Part model, mm, in its own coordinate system. Give positions to 0.01 mm unless a question says otherwise; leave off trailing zeros. Order: outer loops, then holes, each group sorted by start corner. A loop starts at its lowest first (then second) coordinate and runs counter-clockwise, first axis right, second up.
1. Slice it at A-A on y = 44.45. List the corners of the cut face in (x, z).
2. Slice it at C-C on z = 11. Give the number of separate pieces and of enclosed holes in the cut face, and give its area (3 significant figures).
3. Probe line 1 (Y direction, x = 44.45, z = 3.75); line 2 (Y direction, x = 25.4, z = 7.75); line 3 (Y direction, x = 46, z = 6.25). List the from-to ranges inside material, lowest first.
4. Slice it at B-B on x = 25.4. List the corners of the cut face in (y, z), and give its area (3 significant figures).
5. Mould opens along Y. For faces 1 (the cylindrical face through (17.375, 6.424, 6.439)), 2 (the flat face through (0, 25, 6)), 3 (the flat face through (25, 0, 6)) say: +Y half, -Y half, draft (parallel to the pull), parting line (faces both ways), or undercut.
from build123d import *

# Parameters (mm, degrees)
SKETCH1_W           = 50.8
SKETCH1_H           = 50.8
BOSS_EXTRUDE1_DEPTH = 12.7
SKETCH2_R           = 7.62
CUT_EXTRUDE1_DEPTH  = 13.7
SKETCH3_R           = 4.064
CUT_EXTRUDE2_DEPTH  = 13.7
SKETCH4_R           = 1.6764
CUT_EXTRUDE3_DEPTH  = 13.7


with BuildPart() as part:
    # Sketch1 → Boss-Extrude1 (new body)
    with BuildSketch(Plane.XY):
        with Locations((25.4, 25.4)):
            Rectangle(SKETCH1_W, SKETCH1_H)
    extrude(amount=BOSS_EXTRUDE1_DEPTH)

    # Sketch2 → Cut-Extrude1 (cut, through all)
    with BuildSketch(Plane.XY.offset(12.7)):
        with Locations((25.4, 25.4)):
            Circle(SKETCH2_R)
    extrude(amount=-CUT_EXTRUDE1_DEPTH, mode=Mode.SUBTRACT)

    # Sketch3 → Cut-Extrude2 (cut, through all)
    with BuildSketch(Plane.XY.offset(12.7)):
        with Locations((6.35, 44.45)):
            Circle(SKETCH3_R)
        with Locations((6.35, 6.35)):
            Circle(SKETCH3_R)
        with Locations((44.45, 44.45)):
            Circle(SKETCH3_R)
        with Locations((44.45, 6.35)):
            Circle(SKETCH3_R)
    extrude(amount=-CUT_EXTRUDE2_DEPTH, mode=Mode.SUBTRACT)

    # Sketch4 → Cut-Extrude3 (cut, through all)
    with BuildSketch(Plane.XY.offset(12.7)):
        with Locations((19.05, 44.45)):
            Circle(SKETCH4_R)
        with Locations((31.75, 44.45)):
            Circle(SKETCH4_R)
        with Locations((19.05, 6.35)):
            Circle(SKETCH4_R)
        with Locations((31.75, 6.35)):
            Circle(SKETCH4_R)
    extrude(amount=-CUT_EXTRUDE3_DEPTH, mode=Mode.SUBTRACT)


solid = part.part
Data:
1. outline: (0, 0) - (2.29, 0) - (2.29, 12.7) - (0, 12.7) - close; (10.41, 0) - (17.37, 0) - (17.37, 12.7) - (10.41, 12.7) - close; (20.73, 0) - (30.07, 0) - (30.07, 12.7) - (20.73, 12.7) - close; (33.43, 0) - (40.39, 0) - (40.39, 12.7) - (33.43, 12.7) - close; (48.51, 0) - (50.8, 0) - (50.8, 12.7) - (48.51, 12.7) - close
2. separate pieces: 1
2. enclosed holes: 9
2. area: 2,160 mm2
3. line 1: y = 0 to 2.29, 10.41 to 40.39, 48.51 to 50.8
3. line 2: y = 0 to 17.78, 33.02 to 50.8
3. line 3: y = 0 to 2.59, 10.11 to 40.69, 48.21 to 50.8
4. outline: (0, 0) - (17.78, 0) - (17.78, 12.7) - (0, 12.7) - close; (33.02, 0) - (50.8, 0) - (50.8, 12.7) - (33.02, 12.7) - close
4. area: 452 mm2
5. face 1: undercut
5. face 2: draft
5. face 3: -Y half
